Geometry: final body of the model. Coordinates: model frame, mm. Round coordinates to 2 decimals unless told otherwise and drop trailing zeros. Loops run counter-clockwise (first coordinate to the right, second up) from the corner with the lowest first, then second, coordinate; pieces in that order, holes last. Notation, with made-up numbers: (-20.75, 64.5) - (23.25, 64.5) arc R17 ccw to (23.25, 80.5) - close; hole circle Ø9 at (-26.5, -31). An arc over 180 degrees is marked (long way). Return JSON: item names as keys, results as strings. Group by question number.
1. Material intervals for probe 1 along Y at (x, z) = (0, -4.5); probe 2 along Y at (x, z) = (0, 258); probe 3 along Z at (x, y) = (-17, 1.5), sorted ascending.
2. Section A-A on y = -64.5. Return loops of the section in (x, z), and give its area (3 significant figures).
3. Section B-B on z = 169. Return loops of the section in (x, y), and give its area (3 significant figures).
4. First-contact query: pin 1 Ø12 at (x, z) = (7, 258.5) entering from -Y; pin 2 Ø1.1 at (x, z) = (-28.5, 72) entering from -Y; pin 3 Ø6.5 at (x, z) = (-27, -11.5) entering from +Y. Flat tips, straight axial feed; report the tip coordinate or a pass-through.
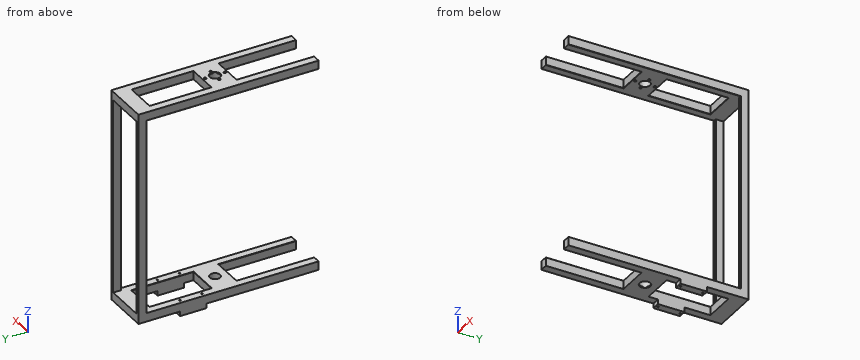
from build123d import *

# Parameters (mm, degrees)
BOSS_EXTRUDE1_START      = -8
SKETCH1_W                = 60
SKETCH1_H                = 230
BOSS_EXTRUDE1_DEPTH      = 11
CUT_EXTRUDE1_DEPTH       = 120.117588961
CUT_EXTRUDE1_DEPTH_BACK  = 120.117588961
SKETCH2_W                = 40
SKETCH2_H                = 99
CUT_EXTRUDE2_DEPTH       = 120.117588961
CUT_EXTRUDE2_DEPTH_BACK  = 120.117588961
SKETCH3_W                = 40
SKETCH3_H                = 79
SKETCH4_W                = 60
SKETCH4_H                = 230
BOSS_EXTRUDE3_DEPTH      = 11
CUT_EXTRUDE3_DEPTH       = 297.373497466
CUT_EXTRUDE3_DEPTH_BACK  = 297.373497466
SKETCH6_W                = 40
SKETCH6_H                = 79
CUT_EXTRUDE4_DEPTH       = 287.33066549
CUT_EXTRUDE4_DEPTH_BACK  = 287.33066549
SKETCH7_W                = 40
SKETCH7_H                = 99
SKETCH8_W                = 4
SKETCH8_H                = 10
BOSS_EXTRUDE4_DEPTH      = 249.5
CUT_EXTRUDE13_DEPTH      = 287.33066549
CUT_EXTRUDE13_DEPTH_BACK = 287.33066549
SKETCH9_R                = 6.5
CUT_EXTRUDE15_START      = -10
SKETCH13_R               = 7
CUT_EXTRUDE15_DEPTH      = 1
SKETCH14_R               = 7
CUT_EXTRUDE16_DEPTH      = 1
CUT_EXTRUDE17_REACH      = 298.373
SKETCH15_R               = 1.6
SKETCH17_W               = 10
SKETCH17_H               = 34
BOSS_EXTRUDE5_DEPTH      = 6
CUT_EXTRUDE18_REACH      = 303.88
SKETCH18_R               = 1
CHAMFER1_SIZE            = 0.3
CHAMFER2_SIZE            = 0.3
CHAMFER3_SIZE            = 0.3
CHAMFER4_SIZE            = 0.3
CHAMFER5_SIZE            = 0.3


with BuildPart() as part:
    # Sketch1 → Boss-Extrude1 (new body)
    with BuildSketch(Plane.XY.offset(BOSS_EXTRUDE1_START)):
        Rectangle(SKETCH1_W, SKETCH1_H)
    extrude(amount=BOSS_EXTRUDE1_DEPTH)

    # Sketch2 → Cut-Extrude1 (cut, two sides: drawn at the far end of the back side and taken through both)
    with BuildSketch(Plane.XY.offset(-CUT_EXTRUDE1_DEPTH_BACK)):
        with Locations((0, -65.5)):
            Rectangle(SKETCH2_W, SKETCH2_H)
    extrude(amount=CUT_EXTRUDE1_DEPTH + CUT_EXTRUDE1_DEPTH_BACK, mode=Mode.SUBTRACT)

    # Sketch3 → Cut-Extrude2 (cut, two sides: drawn at the far end of the back side and taken through both)
    with BuildSketch(Plane.XY.offset(-CUT_EXTRUDE2_DEPTH_BACK)):
        with Locations((0, 55.5)):
            Rectangle(SKETCH3_W, SKETCH3_H)
    extrude(amount=CUT_EXTRUDE2_DEPTH + CUT_EXTRUDE2_DEPTH_BACK, mode=Mode.SUBTRACT)



with BuildPart() as body_2:
    # Sketch4 → Boss-Extrude3 (new body)
    with BuildSketch(Plane.XY.offset(252.5)):
        Rectangle(SKETCH4_W, SKETCH4_H)
    extrude(amount=BOSS_EXTRUDE3_DEPTH)

    # Sketch6 → Cut-Extrude3 (cut, two sides: drawn at the far end of the back side and taken through both)
    with BuildSketch(Plane.XY.offset(263.5).offset(-CUT_EXTRUDE3_DEPTH_BACK)):
        with Locations((0, 55.5)):
            Rectangle(SKETCH6_W, SKETCH6_H)
    extrude(amount=CUT_EXTRUDE3_DEPTH + CUT_EXTRUDE3_DEPTH_BACK, mode=Mode.SUBTRACT)

    # Sketch7 → Cut-Extrude4 (cut, two sides: drawn at the far end of the back side and taken through both)
    with BuildSketch(Plane.XY.offset(252.5).offset(-CUT_EXTRUDE4_DEPTH_BACK)):
        with Locations((0, -65.5)):
            Rectangle(SKETCH7_W, SKETCH7_H)
    extrude(amount=CUT_EXTRUDE4_DEPTH + CUT_EXTRUDE4_DEPTH_BACK, mode=Mode.SUBTRACT)


with BuildPart() as part_1:
    add(part.part)

    add(body_2.part)  # Boss-Extrude4 merges body 2
    # Sketch8 → Boss-Extrude4 (add)
    with BuildSketch(Plane.XY.offset(3)):
        with Locations((-28, 110)):
            Rectangle(SKETCH8_W, SKETCH8_H)
        with Locations((28, 110)):
            Rectangle(SKETCH8_W, SKETCH8_H)
    extrude(amount=BOSS_EXTRUDE4_DEPTH)

    # Sketch9 → Cut-Extrude13 (cut, two sides: drawn at the far end of the back side and taken through both)
    with BuildSketch(Plane.XY.offset(252.5).offset(-CUT_EXTRUDE13_DEPTH_BACK)):
        with Locations(Location((0, 0, 0), (0, 0, 180))):
            Circle(SKETCH9_R)
    extrude(amount=CUT_EXTRUDE13_DEPTH + CUT_EXTRUDE13_DEPTH_BACK, mode=Mode.SUBTRACT)

    # Sketch13 → Cut-Extrude15 (cut)
    with BuildSketch(Plane(origin=(0, 0, 252.5), x_dir=(-1, 0, 0), z_dir=(0, 0, -1)).offset(CUT_EXTRUDE15_START)):
        Circle(SKETCH13_R)
    extrude(amount=-CUT_EXTRUDE15_DEPTH, mode=Mode.SUBTRACT)

    # Sketch14 → Cut-Extrude16 (cut)
    with BuildSketch(Plane(origin=(0, 0, -8), x_dir=(-1, 0, 0), z_dir=(0, 0, -1))):
        Circle(SKETCH14_R)
    extrude(amount=-CUT_EXTRUDE16_DEPTH, mode=Mode.SUBTRACT)

    # Sketch15 → Cut-Extrude17 (cut, up to next)
    with BuildSketch(Plane.XY.offset(263.5), mode=Mode.PRIVATE) as cut_extrude17_sk1:
        with Locations((9.5, 0)):
            Circle(SKETCH15_R)
    cut_extrude17_tool1 = extrude(cut_extrude17_sk1.sketch, amount=-CUT_EXTRUDE17_REACH, mode=Mode.PRIVATE) & part_1.part
    # Sketch15 → Cut-Extrude17 (cut, up to next)
    with BuildSketch(Plane.XY.offset(263.5), mode=Mode.PRIVATE) as cut_extrude17_sk2:
        with Locations(Location((-9.5, 0, 0), (0, 0, 180))):
            Circle(SKETCH15_R)
    cut_extrude17_tool2 = extrude(cut_extrude17_sk2.sketch, amount=-CUT_EXTRUDE17_REACH, mode=Mode.PRIVATE) & part_1.part
    # Sketch15 → Cut-Extrude17 (cut, up to next)
    with BuildSketch(Plane.XY.offset(263.5), mode=Mode.PRIVATE) as cut_extrude17_sk3:
        with Locations((0, 12.5)):
            Circle(SKETCH15_R)
    cut_extrude17_tool3 = extrude(cut_extrude17_sk3.sketch, amount=-CUT_EXTRUDE17_REACH, mode=Mode.PRIVATE) & part_1.part
    # Sketch15 → Cut-Extrude17 (cut, up to next)
    with BuildSketch(Plane.XY.offset(263.5), mode=Mode.PRIVATE) as cut_extrude17_sk4:
        with Locations(Location((0, -12.5, 0), (0, 0, 180))):
            Circle(SKETCH15_R)
    cut_extrude17_tool4 = extrude(cut_extrude17_sk4.sketch, amount=-CUT_EXTRUDE17_REACH, mode=Mode.PRIVATE) & part_1.part
    add(cut_extrude17_tool1.solids().sort_by_distance((9.5, 0, 263.5))[0], mode=Mode.SUBTRACT)
    add(cut_extrude17_tool2.solids().sort_by_distance((-9.5, 0, 263.5))[0], mode=Mode.SUBTRACT)
    add(cut_extrude17_tool3.solids().sort_by_distance((0, 12.5, 263.5))[0], mode=Mode.SUBTRACT)
    add(cut_extrude17_tool4.solids().sort_by_distance((0, -12.5, 263.5))[0], mode=Mode.SUBTRACT)

    # Sketch17 → Boss-Extrude5 (add)
    with BuildSketch(Plane(origin=(0, 0, -8), x_dir=(-1, 0, 0), z_dir=(0, 0, -1))):
        with Locations((25, 45)):
            Rectangle(SKETCH17_W, SKETCH17_H)
        with Locations((-25, 45)):
            Rectangle(SKETCH17_W, SKETCH17_H)
    extrude(amount=BOSS_EXTRUDE5_DEPTH)

    # Sketch18 → Cut-Extrude18 (cut, up to next)
    with BuildSketch(Plane(origin=(0, 0, -14), x_dir=(-1, 0, 0), z_dir=(0, 0, -1)), mode=Mode.PRIVATE) as cut_extrude18_sk1:
        with Locations((-25, 59.2)):
            Circle(SKETCH18_R)
    cut_extrude18_tool1 = extrude(cut_extrude18_sk1.sketch, amount=-CUT_EXTRUDE18_REACH, mode=Mode.PRIVATE) & part_1.part
    # Sketch18 → Cut-Extrude18 (cut, up to next)
    with BuildSketch(Plane(origin=(0, 0, -14), x_dir=(-1, 0, 0), z_dir=(0, 0, -1)), mode=Mode.PRIVATE) as cut_extrude18_sk2:
        with Locations((-25, 31)):
            Circle(SKETCH18_R)
    cut_extrude18_tool2 = extrude(cut_extrude18_sk2.sketch, amount=-CUT_EXTRUDE18_REACH, mode=Mode.PRIVATE) & part_1.part
    # Sketch18 → Cut-Extrude18 (cut, up to next)
    with BuildSketch(Plane(origin=(0, 0, -14), x_dir=(-1, 0, 0), z_dir=(0, 0, -1)), mode=Mode.PRIVATE) as cut_extrude18_sk3:
        with Locations((25, 59.2)):
            Circle(SKETCH18_R)
    cut_extrude18_tool3 = extrude(cut_extrude18_sk3.sketch, amount=-CUT_EXTRUDE18_REACH, mode=Mode.PRIVATE) & part_1.part
    # Sketch18 → Cut-Extrude18 (cut, up to next)
    with BuildSketch(Plane(origin=(0, 0, -14), x_dir=(-1, 0, 0), z_dir=(0, 0, -1)), mode=Mode.PRIVATE) as cut_extrude18_sk4:
        with Locations((25, 31)):
            Circle(SKETCH18_R)
    cut_extrude18_tool4 = extrude(cut_extrude18_sk4.sketch, amount=-CUT_EXTRUDE18_REACH, mode=Mode.PRIVATE) & part_1.part
    add(cut_extrude18_tool1.solids().sort_by_distance((25, 59.2, -14))[0], mode=Mode.SUBTRACT)
    add(cut_extrude18_tool2.solids().sort_by_distance((25, 31, -14))[0], mode=Mode.SUBTRACT)
    add(cut_extrude18_tool3.solids().sort_by_distance((-25, 59.2, -14))[0], mode=Mode.SUBTRACT)
    add(cut_extrude18_tool4.solids().sort_by_distance((-25, 31, -14))[0], mode=Mode.SUBTRACT)

    # Chamfer1
    chamfer1_edges = [part_1.edges().sort_by_distance(p)[0] for p in [
        (-30, -5, 252.5),
    ]]
    chamfer(chamfer1_edges, length=CHAMFER1_SIZE)

    # Chamfer2
    chamfer2_edges = [part_1.edges().sort_by_distance(p)[0] for p in [
        (30, -5, 252.5),
    ]]
    chamfer(chamfer2_edges, length=CHAMFER2_SIZE)

    # Chamfer3
    chamfer3_edges = [part_1.edges().sort_by_distance(p)[0] for p in [
        (-26, 105, 127.75),
        (26, 105, 127.75),
    ]]
    chamfer(chamfer3_edges, length=CHAMFER3_SIZE)

    # Chamfer4
    chamfer4_edges = [part_1.edges().sort_by_distance(p)[0] for p in [
        (-20, -65.5, 3),
        (20, -65.5, 3),
        (0, -16, 3),
        (20, 55.5, 3),
        (0, 95, 3),
        (-20, 55.5, 3),
        (0, 16, 3),
    ]]
    chamfer(chamfer4_edges, length=CHAMFER4_SIZE)

    # Chamfer5
    chamfer5_edges = [part_1.edges().sort_by_distance(p)[0] for p in [
        (20, -65.5, 252.5),
        (0, -16, 252.5),
        (-20, -65.5, 252.5),
        (20, 55.5, 252.5),
        (0, 16, 252.5),
        (-20, 55.5, 252.5),
        (0, 95, 252.5),
    ]]
    chamfer(chamfer5_edges, length=CHAMFER5_SIZE)


solid = part_1.part
Taken from the geometry:
{
 "1": {"probe 1": "-16 to -6.5, 6.5 to 16, 95 to 115", "probe 2": "-16 to -14.1, -10.9 to -6.5, 6.5 to 10.9, 14.1 to 16, 95 to 115", "probe 3": "-8 to 3, 252.5 to 263.5"},
 "2": {"outline": "(-30, -8) - (-20, -8) - (-20, 2.7) - (-20.3, 3) - (-30, 3) - close; (-30, 252.8) - (-29.7, 252.5) - (-20.3, 252.5) - (-20, 252.8) - (-20, 263.5) - (-30, 263.5) - close; (20, -8) - (30, -8) - (30, 3) - (20.3, 3) - (20, 2.7) - close; (20, 252.8) - (20.3, 252.5) - (29.7, 252.5) - (30, 252.8) - (30, 263.5) - (20, 263.5) - close", "area": "440 mm2"},
 "3": {"outline": "(-30, 105) - (-26.3, 105) - (-26, 105.3) - (-26, 115) - (-30, 115) - close; (26, 105.3) - (26.3, 105) - (30, 105) - (30, 115) - (26, 115) - close", "area": "79.9 mm2"},
 "4": {"pin 1": "y = -16", "pin 2": "y = 105", "pin 3": "y = 62"}
}
